Input: part model. Units: mm. Frame: model coordinates. Face numbers are marked on the shaded views. A direction names the side the tool comes from. Give positions to 0.01 mm unless a question says otherwise; leave off trailing zeros. Return JSON: item names as keys, results as strings. Group by question number.
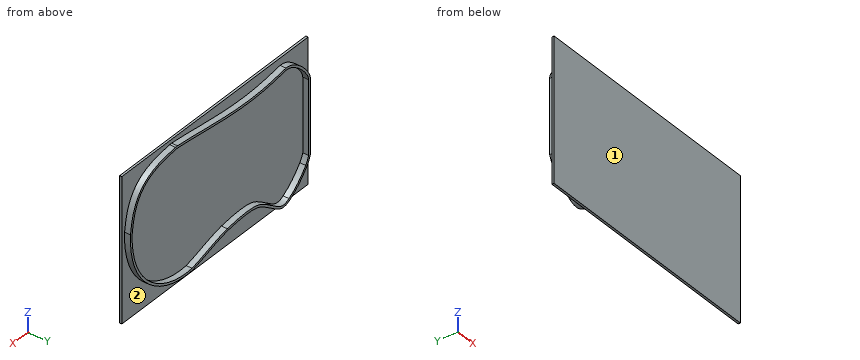
```python
from build123d import *

# Parameters (mm, degrees)
BOSS_EXTRUDE2_DEPTH = 4
SKETCH3_W           = 162.713811117
SKETCH3_H           = 96.815600969
BOSS_EXTRUDE3_DEPTH = 1.5


with BuildPart() as part:
    # Sketch2 → Boss-Extrude2 (new body)
    with BuildSketch(Plane(origin=(0, 0, 0), x_dir=(1, 0, 0), z_dir=(0, 1, 0))):
        with BuildLine():
            Line((-78.157135648, 35.933017955), (-78.157135648, -14.112200016))
            add(Edge.make_bspline(
                [(-78.157135648, -14.112200016), (-78.155939648, -14.752373068), (-77.91728619, -15.977732307), (-77.067841768, -17.98284043), (-75.853766997, -20.009770375), (-73.882725179, -22.698478403), (-70.990105914, -25.858420252), (-67.409604046, -28.950378503), (-64.099125185, -31.13485728), (-61.237861598, -32.390367883), (-59.243018884, -32.778941146), (-57.84210102, -32.875591912), (-57.21182785, -32.900669531), (-56.88815566, -32.920328572)],
                knots=[0.000409109, 0.000409109, 0.000409109, 0.000409109, 0.062842692, 0.125276275, 0.187709857, 0.25014344, 0.375010605, 0.499877771, 0.624744936, 0.749612101, 0.874479267, 0.936912849, 0.999346432, 0.999346432, 0.999346432, 0.999346432], degree=3))
            add(Edge.make_bspline(
                [(-56.88815566, -32.920328572), (-56.642696558, -32.89075012), (-56.160280632, -32.83055745), (-55.130884334, -32.690361106), (-53.775402575, -32.490990423), (-52.023319465, -32.222109613), (-49.529202359, -31.839803624), (-46.118946018, -31.34265718), (-41.582935401, -30.787201605), (-36.628570251, -30.3313494), (-29.499663542, -29.915818278), (-19.674874473, -29.844145156), (-6.636878998, -30.578186936), (5.085601081, -31.774869617), (14.875722867, -32.919022634), (22.392678178, -33.800910905), (30.053166384, -34.637100414), (35.270389761, -35.105189919), (37.869497862, -35.297508229)],
                knots=[-0.001372968, -0.001372968, -0.001372968, -0.001372968, 0.014272852, 0.029918673, 0.061210313, 0.092501954, 0.123793594, 0.186376875, 0.248960156, 0.311543437, 0.374126718, 0.49929328, 0.624459842, 0.749626404, 0.812209685, 0.874792966, 0.937376247, 0.999959528, 0.999959528, 0.999959528, 0.999959528], degree=3))
            ThreePointArc((37.869497862, -35.297508229), (38.735359767, -35.294029869), (39.597461801, -35.21335137))
            add(Edge.make_bspline(
                [(39.597461801, -35.21335137), (41.139767175, -35.04904175), (44.235594855, -34.704530206), (50.30182099, -33.820891122), (57.45023856, -32.130120831), (64.799112885, -28.716371013), (70.578195113, -23.811075447), (73.965626007, -18.700600273), (75.883187129, -14.305672198), (76.967229357, -10.961986186), (77.747932295, -7.691449122), (78.199718827, -5.145010951), (78.480402727, -3.296584904), (78.661323244, -2.03081469), (78.823959845, -0.900875926), (78.927618693, -0.280644372), (78.981646775, 0.045841454)],
                knots=[-8.5538e-05, -8.5538e-05, -8.5538e-05, -8.5538e-05, 0.063427598, 0.126940734, 0.253967006, 0.380993278, 0.50801955, 0.635045822, 0.698558958, 0.762072094, 0.82558523, 0.889098367, 0.920854935, 0.952611503, 0.984368071, 1.016124639, 1.016124639, 1.016124639, 1.016124639], degree=3))
            add(Edge.make_bspline(
                [(78.981646775, 0.045841454), (79.027094782, 1.179674429), (79.064720926, 3.473913783), (78.944393791, 6.769688051), (78.658660296, 9.974948397), (78.064183944, 14.11691568), (76.934054174, 19.032604235), (74.364574026, 26.339835799), (69.843932164, 34.39440102), (62.712031102, 42.254317161), (54.262624742, 48.235080745), (44.879874513, 52.267066292), (34.952870186, 54.2885898), (28.210881807, 54.235085369), (24.886864743, 53.860071186)],
                knots=[-0.00040736, -0.00040736, -0.00040736, -0.00040736, 0.030879521, 0.062166401, 0.093453282, 0.124740163, 0.187313924, 0.249887685, 0.375035208, 0.50018273, 0.625330253, 0.750477775, 0.875625298, 1.00077282, 1.00077282, 1.00077282, 1.00077282], degree=3))
            add(Edge.make_bspline(
                [(24.886864743, 53.860071186), (22.283887479, 53.234934331), (17.122333316, 51.770006392), (6.978810179, 48.483475597), (-0.62058189, 46.171110399), (-5.82261915, 45.177242661)],
                knots=[-0.001280714, -0.001280714, -0.001280714, -0.001280714, 0.24771449, 0.496709693, 0.9947001, 0.9947001, 0.9947001, 0.9947001], degree=3))
            add(Edge.make_bspline(
                [(-5.82261915, 45.177242661), (-6.846271695, 45.033725935), (-8.877911438, 44.761027761), (-13.088195507, 44.259306095), (-18.264324114, 43.792662786), (-23.901821518, 43.633821839), (-28.702631501, 43.985910311), (-32.652338295, 44.908532737), (-35.447699325, 46.177033317), (-37.648428, 47.515223041), (-39.36186509, 48.682387067), (-40.924837411, 49.79297126), (-42.29202762, 50.749624529), (-43.050520295, 51.26512862), (-43.422492414, 51.515145542)],
                knots=[0.000305139, 0.000305139, 0.000305139, 0.000305139, 0.063047866, 0.125790592, 0.251276044, 0.376761496, 0.502246948, 0.627732401, 0.753217853, 0.815960579, 0.878703305, 0.941446031, 0.972817394, 1.004188757, 1.004188757, 1.004188757, 1.004188757], degree=3))
            add(Edge.make_bspline(
                [(-43.422492414, 51.515145542), (-43.678616345, 51.691810139), (-44.195843457, 52.052612418), (-45.168447607, 52.746174672), (-46.308029686, 53.571366973), (-47.576953364, 54.472121728), (-49.172650358, 55.533487702), (-51.044076917, 56.564817563), (-53.214706641, 57.25190115), (-55.319518496, 57.36517967), (-56.956778648, 57.053303598), (-58.147723245, 56.650637672), (-58.968859533, 56.298465061), (-59.57079354, 55.992027065), (-60.005881741, 55.748275575), (-60.18615305, 55.640555889), (-60.280341084, 55.583909473)],
                knots=[-0.002293809, -0.002293809, -0.002293809, -0.002293809, 0.029244556, 0.060782921, 0.123859651, 0.186936381, 0.250013112, 0.376166572, 0.502320033, 0.628473494, 0.754626954, 0.817703684, 0.880780415, 0.943857145, 0.97539551, 1.006933875, 1.006933875, 1.006933875, 1.006933875], degree=3))
            add(Edge.make_bspline(
                [(-60.280341084, 55.583909473), (-60.714952444, 55.32966131), (-61.58200578, 54.800998059), (-63.22221391, 53.718688993), (-65.910533435, 51.737250649), (-69.243121764, 48.741031753), (-72.024440988, 45.692878732), (-73.73920341, 43.627948753), (-74.665747867, 42.475614869), (-75.104907594, 41.920162476), (-75.326466464, 41.639029179)],
                knots=[0.000426683, 0.000426683, 0.000426683, 0.000426683, 0.06326809, 0.126109496, 0.251792309, 0.503157934, 0.75452356, 0.880206373, 0.943047779, 1.005889185, 1.005889185, 1.005889185, 1.005889185], degree=3))
            add(Edge.make_bspline(
                [(-75.326466464, 41.639029179), (-75.91997327, 40.746000391), (-77.006363229, 38.87012428), (-77.815024814, 36.931350625), (-78.157135648, 35.933017955)],
                knots=[0.49954614, 0.49954614, 0.49954614, 0.49954614, 0.499770438, 0.499994735, 0.499994735, 0.499994735, 0.499994735], degree=3))
        make_face()
        with BuildLine():
            Line((-76.657135648, 35.679066848), (-76.657131969, -14.112200006))
            add(Edge.make_bspline(
                [(-76.657131969, -14.112200006), (-76.656531466, -14.340940611), (-76.615532486, -14.780598422), (-76.365572342, -15.779633829), (-75.747022441, -17.26132375), (-74.637885805, -19.124336874), (-72.785033195, -21.666520065), (-70.027170511, -24.69605914), (-66.602535352, -27.672706005), (-63.476928114, -29.755963329), (-60.874171764, -30.916444124), (-58.823492797, -31.343417769), (-57.575149509, -31.379323699), (-56.935294504, -31.415052584)],
                knots=[0.000537135, 0.000537135, 0.000537135, 0.000537135, 0.031486368, 0.0624356, 0.124334065, 0.186232529, 0.248130994, 0.371927923, 0.495724853, 0.619521782, 0.743318712, 0.867115641, 0.99091257, 0.99091257, 0.99091257, 0.99091257], degree=3))
            add(Edge.make_bspline(
                [(-56.935294504, -31.415052584), (-56.694661939, -31.385667933), (-56.223603705, -31.325866144), (-55.203470476, -31.185340461), (-53.856324583, -30.986089165), (-52.101912742, -30.716485052), (-49.596504581, -30.333088531), (-46.159583081, -29.834426322), (-41.581560568, -29.27829752), (-36.581457935, -28.823458861), (-29.390698582, -28.411647175), (-19.497861615, -28.34813345), (-6.407460838, -29.092198199), (7.671085742, -30.53241701), (20.045487362, -32.035993294), (30.203761894, -33.14440123), (35.375718345, -33.608610084), (37.954323811, -33.799682751)],
                knots=[0.001496116, 0.001496116, 0.001496116, 0.001496116, 0.017093844, 0.032691572, 0.063887028, 0.095082483, 0.126277939, 0.18866885, 0.251059761, 0.313450672, 0.375841584, 0.500623406, 0.625405228, 0.750187051, 0.874968873, 0.937359784, 0.999750695, 0.999750695, 0.999750695, 0.999750695], degree=3))
            ThreePointArc((37.954323811, -33.799682751), (38.685754809, -33.794634443), (39.413826008, -33.724426748))
            add(Edge.make_bspline(
                [(39.413826008, -33.724426748), (40.941587091, -33.561666605), (44.016933216, -33.219818338), (49.974357897, -32.353936258), (56.920589371, -30.71373603), (63.928940419, -27.467086873), (69.37640321, -22.871797273), (72.592452605, -18.066629926), (74.435319216, -13.886326636), (75.48738516, -10.677838243), (76.252417838, -7.512200065), (76.699454408, -5.023141593), (76.979420749, -3.19383512), (77.160428463, -1.932130727), (77.326847127, -0.768127182), (77.43119015, -0.135396957), (77.486499649, 0.198499569)],
                knots=[-0.000425037, -0.000425037, -0.000425037, -0.000425037, 0.062921118, 0.126267272, 0.25295958, 0.379651889, 0.506344198, 0.633036506, 0.696382661, 0.759728815, 0.823074969, 0.886421123, 0.918094201, 0.949767278, 0.981440355, 1.013113432, 1.013113432, 1.013113432, 1.013113432], degree=3))
            add(Edge.make_bspline(
                [(77.486499649, 0.198499569), (77.529376832, 1.304965595), (77.563148654, 3.54640861), (77.441718254, 6.750377683), (77.160012317, 9.869265522), (76.577911195, 13.891943853), (75.476896458, 18.658811745), (72.98279324, 25.733467023), (68.609003035, 33.517419822), (61.718308835, 41.112614632), (53.552963068, 46.899058336), (44.478248309, 50.80844929), (34.878936934, 52.776287746), (28.361333333, 52.735962773), (25.146710313, 52.37977831)],
                knots=[0.000462258, 0.000462258, 0.000462258, 0.000462258, 0.031684846, 0.062907434, 0.094130022, 0.125352611, 0.187797787, 0.250242963, 0.375133316, 0.500023669, 0.624914022, 0.749804375, 0.874694728, 0.999585081, 0.999585081, 0.999585081, 0.999585081], degree=3))
            add(Edge.make_bspline(
                [(25.146710313, 52.37977831), (19.996880057, 51.137756564), (12.46311825, 48.651529878), (2.282936309, 45.485639859), (-2.943523861, 44.200173327), (-5.577592643, 43.696925109)],
                knots=[0.001647883, 0.001647883, 0.001647883, 0.001647883, 0.49875575, 0.747309683, 0.995863617, 0.995863617, 0.995863617, 0.995863617], degree=3))
            add(Edge.make_bspline(
                [(-5.577592643, 43.696925109), (-6.608686649, 43.552365086), (-8.654048562, 43.277286792), (-12.900719679, 42.770558047), (-18.1416297, 42.296463944), (-23.901116409, 42.131322734), (-28.894462751, 42.491806828), (-33.123562317, 43.472784898), (-36.152698653, 44.848626269), (-38.469673728, 46.259294554), (-40.227820016, 47.45749815), (-41.798031425, 48.573285436), (-43.149641227, 49.51893077), (-43.899165402, 50.028194293), (-44.266747833, 50.275260736)],
                knots=[-0.000445954, -0.000445954, -0.000445954, -0.000445954, 0.062356884, 0.125159722, 0.250765398, 0.376371074, 0.50197675, 0.627582426, 0.753188102, 0.81599094, 0.878793778, 0.941596616, 0.972998035, 1.004399454, 1.004399454, 1.004399454, 1.004399454], degree=3))
            add(Edge.make_bspline(
                [(-44.266747833, 50.275260736), (-44.527408356, 50.455054502), (-45.054249251, 50.822434727), (-46.041767018, 51.526583503), (-47.182852187, 52.352899291), (-48.430502857, 53.238394378), (-49.959355128, 54.254926441), (-51.669032297, 55.190671355), (-53.504011998, 55.762856637), (-55.217112111, 55.853610566), (-56.862754072, 55.542492613), (-58.118908127, 55.048422463), (-58.991920159, 54.602781729), (-59.334940415, 54.402109669), (-59.515062385, 54.293781003)],
                knots=[-0.002598924, -0.002598924, -0.002598924, -0.002598924, 0.0289762, 0.060551324, 0.123701572, 0.18685182, 0.250002068, 0.376302564, 0.502603061, 0.628903557, 0.755204053, 0.881504549, 0.944654797, 1.007805046, 1.007805046, 1.007805046, 1.007805046], degree=3))
            add(Edge.make_bspline(
                [(-59.515062385, 54.293781003), (-59.933000678, 54.049286604), (-60.767107189, 53.541199426), (-62.34414566, 52.501351132), (-64.932965719, 50.59560099), (-68.153458432, 47.704906594), (-70.856343693, 44.749408068), (-72.789087262, 42.425042933), (-73.666165752, 41.322178137), (-74.110264621, 40.758884118)],
                knots=[4.7776e-05, 4.7776e-05, 4.7776e-05, 4.7776e-05, 0.062686674, 0.125325571, 0.250603366, 0.501158957, 0.751714547, 0.876992343, 1.002270138, 1.002270138, 1.002270138, 1.002270138], degree=3))
            add(Edge.make_bspline(
                [(-74.110264621, 40.758884118), (-74.638638681, 39.959603427), (-75.611693177, 38.281434426), (-76.343021988, 36.564567869), (-76.657135648, 35.679066848)],
                knots=[0.49955057, 0.49955057, 0.49955057, 0.49955057, 0.499763362, 0.499976154, 0.499976154, 0.499976154, 0.499976154], degree=3))
        make_face(mode=Mode.SUBTRACT)
    extrude(amount=BOSS_EXTRUDE2_DEPTH)

    # Sketch3 → Boss-Extrude3 (add)
    with BuildSketch(Plane.XZ):
        with Locations((0.019032639, -10.611106307)):
            Rectangle(SKETCH3_W, SKETCH3_H)
    extrude(amount=BOSS_EXTRUDE3_DEPTH)


solid = part.part
```
Item 1: Material intervals for line 1 (X direction, y = 0.6, z = -0.5); line 2 (X direction, y = 1.7, z = -42); line 3 (Y direction, x = 41, z = -39), sorted ascending. Write a range as from..to.
Item 2: First-contact query: pin 1 Ø1.5 at (x, z) = (-18, -15.5) entering from +Y; pin 2 Ø3 at (y, z) = (2.5, -35.5) entering from +X. Flat tips, straight axial feed; report the tip coordinate or a pass-through.
Item 3: Reachability of the marked faces 1 and 2 from +Z, -Z, +X, -X, +Y, -Y: full face, straight path, thin tool, end or side. Return the list, or none.
Answer below:
{
 "1": {"line 1": "-78.16..-76.66, 77.5..79", "line 2": "-75.04..-73.12, 60.11..62.43", "line 3": "-1.5..0"},
 "2": {"pin 1": "y = 0", "pin 2": "x = 69.63"},
 "3": {"face 1": "+Z, -Z, +X, -X, -Y", "face 2": "+Y"}
}
